Source: three-view drawing plus pictorial views. Frame: mm from the lowest corner of the part. A direction names the side the tool comes from. Give positions to 0.01 mm unless a question says otherwise; leave off trailing zeros. Loops run counter-clockwise (first coordinate to the right, second up) from the corner with the lowest first, then second, coordinate; pieces in that order, holes last. Notation, with made-up numbers: (36, -26.75) - (50, -26.75) arc R30 cw to (50, -2.75) - close; hole circle Ø2 at (-9.75, 42). An arc over 180 degrees is marked (long way). Answer as a JSON object with one key per item and string values. Group by question number.
(1) Mould query, pull axis X, two halves, no side actions, for the marked faces 1 and 2. Classes: +X half, -X half, draft (parallel to the pull), parting line (faces both ways), or undercut.
(2) Access query for the marked faces 3 and 4. Directions: +Z, -Z, +X, -X, +Y, -Y. A direction counts if a zero-diameter tool reaches every point of the face in a straight line with its end or side. Return the directions, or none.
(3) Pin query (flat end, axial travel): P1, Ø1.2, axis at x = 2.54, z = 17.526, coming from the -Y side; P2, Ø5, axis at x = 10, y = 5.5, coming from the +Z side; P3, Ø5, axis at y = 6, z = 16, coming from the -X side; P4, Ø2, axis at y = 12, z = 3, coming from the -X side. Return the tip coordinate at first contact, or that it passes through.
(4) Section query D-D (z = 13.5). Return loops of the section in (x, y), plus the area to 3 significant figures.
(5) Section query B-B (x = 33.02). Return loops of the section in (y, z).
(6) Material intervals for L1, parallel to Z at x = 40.64, y = 0.5; L2, parallel to Z at x = 2.54, y = 1.65; L3, parallel to Y at x = 31, z = 1.25, sorted ascending.
(7) Section query C-C (y = 6). Return loops of the section in (x, z), plus the area to 3 significant figures.
(8) Section query A-A (z = 2.54). Return loops of the section in (x, y), plus the area to 3 significant figures.
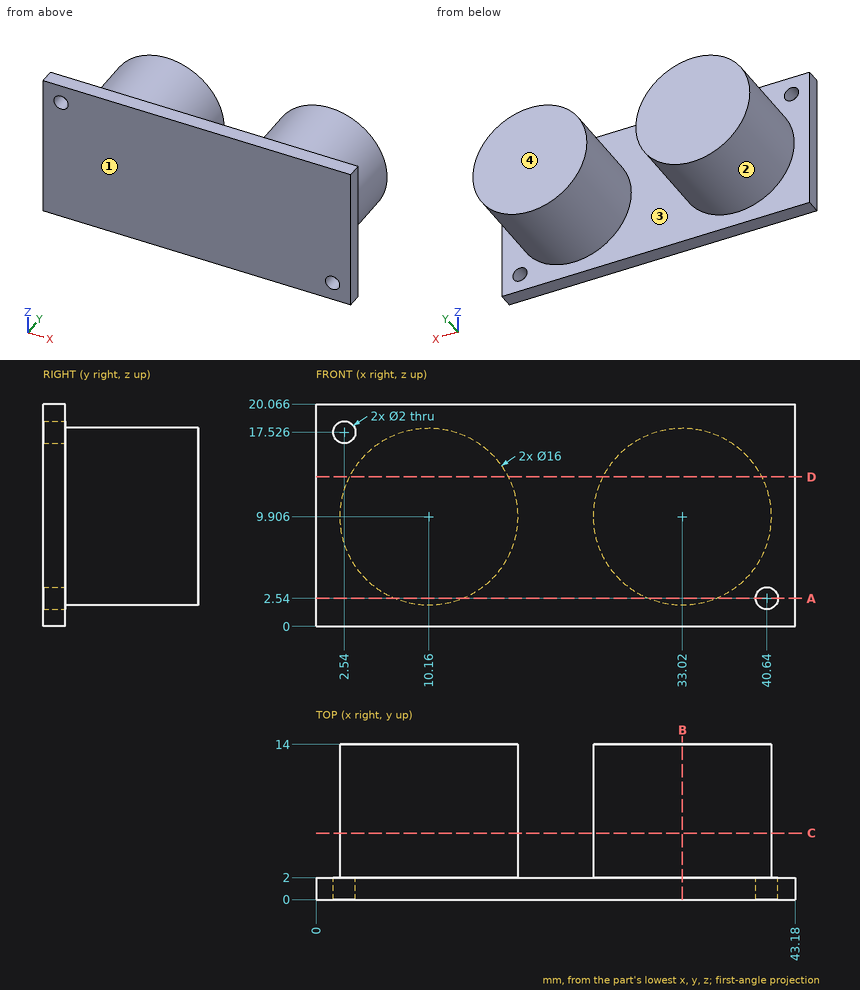
Recorded:
{
 "1": {"face 1": "draft", "face 2": "undercut"},
 "2": {"face 3": "+Y", "face 4": "+Z, -Z, +X, -X, +Y"},
 "3": {"P1": "passes through", "P2": "stops at z = 17.91", "P3": "stops at x = 3.01", "P4": "stops at x = 4.76"},
 "4": {"outline": "(0, 0) - (43.18, 0) - (43.18, 2) - (40.17, 2) - (40.17, 14) - (25.87, 14) - (25.87, 2) - (17.31, 2) - (17.31, 14) - (3.01, 14) - (3.01, 2) - (0, 2) - close", "area": "429 mm^2"},
 "5": {"outline": "(0, 0) - (2, 0) - (2, 1.91) - (14, 1.91) - (14, 17.91) - (2, 17.91) - (2, 20.07) - (0, 20.07) - close"},
 "6": {"L1": "z = 0 to 1.54, 3.54 to 20.07", "L2": "z = 0 to 16.53, 18.53 to 20.07", "L3": "y = 0 to 2"},
 "7": {"outline": "circle Ø16 at (10.16, 9.91); circle Ø16 at (33.02, 9.91)", "area": "402 mm^2"},
 "8": {"outline": "(0, 0) - (39.64, 0) - (39.64, 2) - (36.14, 2) - (36.14, 14) - (29.9, 14) - (29.9, 2) - (13.28, 2) - (13.28, 14) - (7.04, 14) - (7.04, 2) - (0, 2) - close; (41.64, 0) - (43.18, 0) - (43.18, 2) - (41.64, 2) - close", "area": "232 mm^2"}
}
